Model file for the job. Use its own axes, mm. A direction names the side the tool comes from. Coordinates: 2 decimals unless noted, no trailing zeros. Order: outer loops, then holes, each group sorted by start corner. A loop starts at its lowest first (then second) coordinate and runs counter-clockwise, first axis right, second up. Notation, with made-up numbers: (-39, 50) -> (-26, 50) arc R36 cw to (-26, 88) -> close; hole circle Ø4 at (68, 80.25). An arc over 180 degrees is marked (long way). Write item = value, one per line. Start each with the question number.
Q1. Wall check: line 1 (X direction, y = 8, z = -6.25); line 2 (Y direction, x = -21.5, z = -6.5); line 3 (Z direction, x = -10.75, y = 5.75). Give the ranges that are in metal, low to high. Write a range as from..to.
Q2. Cut at D-D, the plane y = 8. List the corners of the cut face in (x, z).
Q3. Cut at A-A, the plane y = 5.25. List the corners of the cut face in (x, z), plus the area to 3 significant figures.
Q4. Flat gauge pins, fed straight in: pin 1 (1.6 mm diameter, centred on y = 5.5, z = -8.5, fed in from +X); pin 2 (1.2 mm diameter, centred on y = 4.5, z = -8, fed in from -X). Where does each tip first touch, or does it go through?
Q5. Cut at B-B, the plane x = 3. List the corners of the cut face in (y, z).
Q6. Cut at C-C, the plane x = -6. List the corners of the cut face in (y, z), plus the area to 3 significant figures.
Q7. 3-axis set-ups, long thin cutter, end or side, ignore diameter. For faces 1 (the face through (-15.193, 4.93, -7.368)), 2 (the face through (-16.595, 5, -8)), 3 (the face through (3.3, 7, -7.1)): which of +Z, -Z, +X, -X, +Y, -Y reach the whole face in a straight line?
Q8. Mould opens along Y. For faces 4 (the face through (-8, 5, -9)), 5 (the face through (-8, 0, -7)), 6 (the face through (3.3, 3, -7.1)) say: +Y half, -Y half, draft (parallel to the pull), parting line (faces both ways), or undercut.
from build123d import *

# Parameters (mm, degrees)
BOSS_EXTRUDE2_DEPTH = 10
SKETCH2_W           = 6.583630945
SKETCH2_H           = 4
SKETCH2_W_2         = 6.583630944
CUT_EXTRUDE1_DEPTH  = 20


with BuildPart() as part:
    # Sketch1 → Boss-Extrude2 (new body)
    with BuildSketch(Plane(origin=(0, 0, 0), x_dir=(1, 0, 0), z_dir=(0, 1, 0))):
        with BuildLine():
            ThreePointArc((-9.797308403, 3.169636963), (-15.292255473, 7.386058148), (-21.897917664, 5.303300859))
            ThreePointArc((-21.897917664, 5.303300859), (-22.958577836, 5.303300859), (-22.958577836, 6.363961031))
            ThreePointArc((-22.958577836, 6.363961031), (-20.038767697, 8.314915793), (-16.594616806, 9))
            Line((-16.594616806, 9), (0, 9))
            ThreePointArc((0, 9), (3.444150891, 8.314915793), (6.363961031, 6.363961031))
            ThreePointArc((6.363961031, 6.363961031), (6.363961031, 5.303300859), (5.303300859, 5.303300859))
            ThreePointArc((5.303300859, 5.303300859), (-1.302361333, 7.386058148), (-6.797308403, 3.169636963))
            ThreePointArc((-6.797308403, 3.169636963), (-7.415063167, 2.287391728), (-8.297308403, 1.669636963))
            ThreePointArc((-8.297308403, 1.669636963), (-9.179553638, 2.287391728), (-9.797308403, 3.169636963))
        make_face()
    extrude(amount=BOSS_EXTRUDE2_DEPTH)

    # Sketch2 → Cut-Extrude1 (cut)
    with BuildSketch(Plane(origin=(0, 0, -9), x_dir=(-1, 0, 0), z_dir=(0, 0, -1))):
        with Locations((-3.291815473, 5)):
            Rectangle(SKETCH2_W, SKETCH2_H)
        with Locations((19.886432278, 5)):
            Rectangle(SKETCH2_W_2, SKETCH2_H)
    extrude(amount=-CUT_EXTRUDE1_DEPTH, mode=Mode.SUBTRACT)


solid = part.part
Here are the results:
q1.line_1 = -23.05..-20.74, -12.45..-4.15, 4.15..6.46
q1.line_2 = 0..3, 7..10
q1.line_3 = -9..-4.7
q2.outline = (-22.96, -6.36) arc R9 ccw to (-16.59, -9) -> (0, -9) arc R9 ccw to (6.36, -6.36) arc R0.75 ccw to (5.3, -5.3) arc R7.5 cw to (-6.8, -3.17) arc R3.1 ccw to (-8.3, -1.67) arc R3.1 ccw to (-9.8, -3.17) arc R7.5 cw to (-21.9, -5.3) arc R0.75 ccw to start
q3.outline = (-16.59, -9) -> (0, -9) -> (0, -7.5) arc R7.5 cw to (-6.8, -3.17) arc R3.1 ccw to (-8.3, -1.67) arc R3.1 ccw to (-9.8, -3.17) arc R7.5 cw to (-16.59, -7.5) -> close
q3.area = 57.3 mm²
q4.pin_1 = 0
q4.pin_2 = -16.59
q5.outline = (0, -8.49) -> (3, -8.49) -> (3, -6.87) -> (0, -6.87) -> close; (7, -8.49) -> (10, -8.49) -> (10, -6.87) -> (7, -6.87) -> close
q6.outline = (0, -9) -> (10, -9) -> (10, -4.5) -> (0, -4.5) -> close
q6.area = 45.0 mm²
q7.face_1 = +Z, +Y, -Y
q7.face_2 = +Z, -Z, -X
q7.face_3 = +Z, -Z, +X
q8.face_4 = draft
q8.face_5 = -Y half
q8.face_6 = undercut
